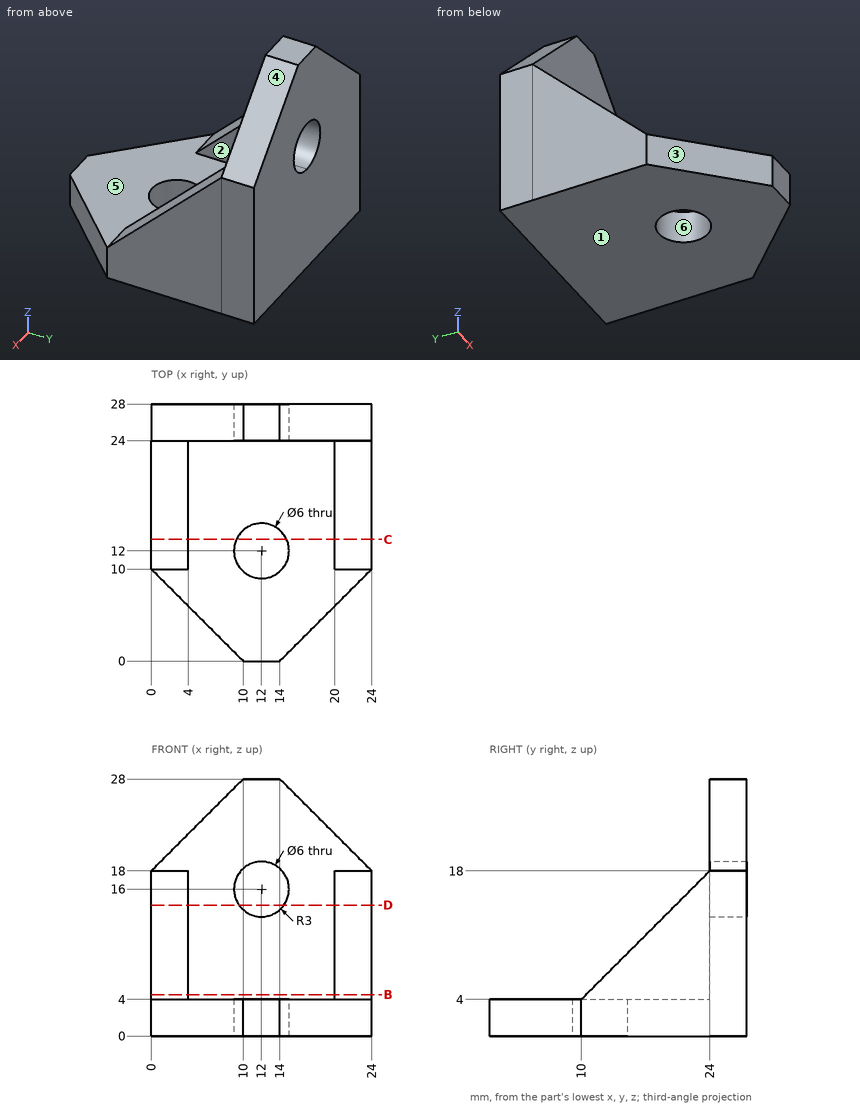
Design review of the part shown in the three views and the two pictorial views. Dimensions are in mm from the part's minimum x, y and z. A direction names the side the tool comes from. Coordinates: 2 decimals unless noted, no trailing zeros. Loops run counter-clockwise (first coordinate to the right, second up) from the corner with the lowest first, then second, coordinate; pieces in that order, holes last.
Q1. The part is to be moulded in two halves that separate along X. For the marked faces 1, 2, 3 and 4, say which applies: +X half, -X half, draft (parallel to the pull), parting line (faces both ways), or undercut.
Reported:
face 1: draft
face 2: undercut
face 3: -X half
face 4: +X half
Q2. We need section D-D on z = 14.25. State the section outline as (x, y) points.
Reported:
outline: (0, 20.25) - (4, 20.25) - (4, 24) - (9.56, 24) - (9.56, 28) - (0, 28) - close; (14.44, 24) - (20, 24) - (20, 20.25) - (24, 20.25) - (24, 28) - (14.44, 28) - close
Q3. For pin 1 (1 mm diameter, centred on x = 2.5, y = 17.5, fed in from +Z), flat-tipped, find the tip position at first contact; note if it passes through.
Reported:
pin 1: stops at z = 12
Q4. To check wall thickness, follow line 1 (Y direction, x = 12, z = 2.35); line 2 (Y direction, x = 9.25, z = 19.25); line 3 (X direction, y = 25, z = 16). State the ranges of each line that lie inside material, in increasing order.
Reported:
line 1: y = 0 to 9, 15 to 28
line 2: y = 24 to 28
line 3: x = 0 to 9, 15 to 24
Q5. We need section B-B on z = 4.5. State the section outline as (x, y) points, and give its area (3 significant figures).
Reported:
outline: (0, 10.5) - (4, 10.5) - (4, 24) - (20, 24) - (20, 10.5) - (24, 10.5) - (24, 28) - (0, 28) - close
area: 204 mm2
Q6. Tool access review of the marked faces 5 and 6: name each direction out of +Z, -Z, +X, -X, +Y, -Y from which nothing blocks a thin tool from reaching the whole face with its end or side.
Reported:
face 5: +Z, -Y
face 6: +Z, -Z
Q7. We need section C-C on y = 13.25. State the section outline as (x, z) points.
Reported:
outline: (0, 0) - (9.27, 0) - (9.27, 4) - (4, 4) - (4, 7.25) - (0, 7.25) - close; (14.73, 0) - (24, 0) - (24, 7.25) - (20, 7.25) - (20, 4) - (14.73, 4) - close
